Design review of the part built by this model. Coordinates are the model's own, in mm. Face numbers are marked on the shaded views. Give positions to 0.01 mm unless a question says otherwise; leave off trailing zeros. Write each loop counter-clockwise with the first axis right and the second up, starting at its lowest first coordinate (ties: lowest second). Pieces come first, ordered by that corner, then holes. Notation, with made-up numbers: (-6.5, -29) -> (10.5, -29) arc R9 cw to (10.5, -24) -> close; hole circle Ø7 at (20, 24). An arc over 180 degrees is marked (long way). Answer as a JSON object with one key per item and string values.
```python
from build123d import *

# Parameters (mm, degrees)
SKETCH1_R           = 75
BOSS_EXTRUDE1_DEPTH = 3
SKETCH2_R           = 75
SKETCH2_R_2         = 72
BOSS_EXTRUDE2_DEPTH = 150
SKETCH3_R           = 5
CUT_EXTRUDE1_DEPTH  = 150


with BuildPart() as part:
    # Sketch1 → Boss-Extrude1 (new body)
    with BuildSketch(Plane.XY):
        Circle(SKETCH1_R)
    extrude(amount=BOSS_EXTRUDE1_DEPTH)

    # Sketch2 → Boss-Extrude2 (add)
    with BuildSketch(Plane.XY.offset(3)):
        Circle(SKETCH2_R)
        Circle(SKETCH2_R_2, mode=Mode.SUBTRACT)
    extrude(amount=BOSS_EXTRUDE2_DEPTH)

    # Sketch3 → Cut-Extrude1 (cut)
    with BuildSketch(Plane.XY.offset(3)):
        with Locations((30, 0)):
            Circle(SKETCH3_R)
        with Locations((-30, 0)):
            Circle(SKETCH3_R)
    extrude(amount=-CUT_EXTRUDE1_DEPTH, mode=Mode.SUBTRACT)


solid = part.part
```
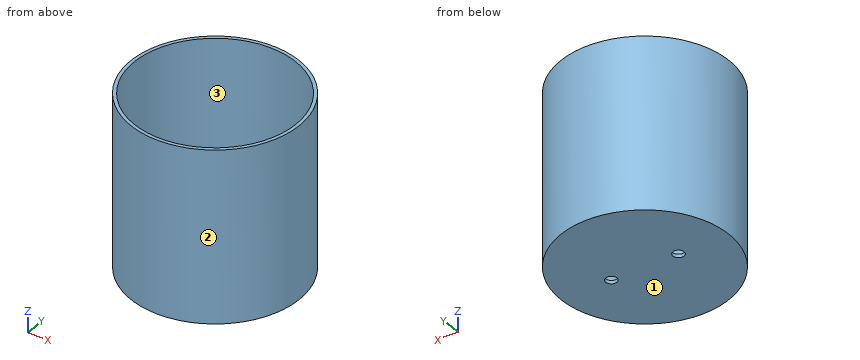
(1) Clearance check with flat-ended pins moving along their axes: pin 1 (2 mm diameter, centred on y = 4, z = 22, fed in from +X); pin 2 (2 mm diameter, centred on x = 56.5, z = 91, fed in from +Y); pin 3 (6 mm diameter, centred on y = 18, z = 61, fed in from -X); pin 4 (6 mm diameter, centred on x = 30, y = 0, fed in from -Z). State where each tip first meets the part, or that it passes through.
Here are the results:
{"pin 1": "stops at x = 74.94", "pin 2": "stops at y = 50.45", "pin 3": "stops at x = -73.48", "pin 4": "passes through"}
(2) For line 1 along Y through (x, z) = (0, 113); line 2 along Z through (x, y) = (17.5, -60.5); line 3 along Y through (x, z) = (3, 32), list the stretches that pass through material, from the lowest coordinate up.
Here are the results:
{"line 1": "y = -75 to -72, 72 to 75", "line 2": "z = 0 to 3", "line 3": "y = -74.94 to -71.94, 71.94 to 74.94"}
(3) The part is to be moulded in two halves that separate along Y. For the marked faces 1, 2 and 3, say which applies: +Y half, -Y half, draft (parallel to the pull), parting line (faces both ways), or undercut.
Here are the results:
{"face 1": "draft", "face 2": "parting line", "face 3": "undercut"}
(4) We need section C-C, the plane y = -62.5. State the section outline as (x, z) points, then the cut area to 3 significant figures.
Here are the results:
{"outline": "(-41.46, 0) -> (41.46, 0) -> (41.46, 153) -> (35.75, 153) -> (35.75, 3) -> (-35.75, 3) -> (-35.75, 153) -> (-41.46, 153) -> close", "area": "1,960 mm²"}
(5) We need section A-A, the plane x = 29. State the section outline as (y, z) points.
Here are the results:
{"outline": "(-69.17, 0) -> (-4.9, 0) -> (-4.9, 3) -> (-65.9, 3) -> (-65.9, 153) -> (-69.17, 153) -> close; (4.9, 0) -> (69.17, 0) -> (69.17, 153) -> (65.9, 153) -> (65.9, 3) -> (4.9, 3) -> close"}
(6) We need section B-B, the plane z = 95.5. State the section outline as (x, y) points.
Here are the results:
{"outline": "circle Ø150 at (0, 0); hole circle Ø144 at (0, 0)"}
(7) We need section D-D, the plane x = 11. State the section outline as (y, z) points, then the cut area to 3 significant figures.
Here are the results:
{"outline": "(-74.19, 0) -> (74.19, 0) -> (74.19, 153) -> (71.15, 153) -> (71.15, 3) -> (-71.15, 3) -> (-71.15, 153) -> (-74.19, 153) -> close", "area": "1,360 mm²"}
